Read the model definition and answer for the solid it produces. Units are mm, in the model's axes. A direction names the side the tool comes from. Coordinates: 2 decimals unless noted, no trailing zeros. Write each loop counter-clockwise with the first axis right and the second up, starting at its lowest first coordinate (ties: lowest second). Pieces come first, ordered by that corner, then holes. Notation, with made-up numbers: (22, 11.25) -> (76, 11.25) arc R18 cw to (76, 32.25) -> close; hole circle Ø11 at (35.5, 32). An arc over 180 degrees is marked (long way). Use CSV: the item, a comma, the result in double quotes.
from build123d import *

# Parameters (mm, degrees)
F0_W           = 400
F0_H           = 400
F1_DEPTH       = 50
F2_R           = 6
F3_DEPTH       = 35
F5_D           = 17
F5_DEPTH       = 53
F5_CBORE_D     = 28
F5_CBORE_DEPTH = 20


with BuildPart() as f1:
    # F0 (on Top) → F1 (new body)
    with BuildSketch(Plane.XY):
        Rectangle(F0_W, F0_H)
    extrude(amount=-F1_DEPTH)

    # F2 (on face) → F3 (cut)
    with BuildSketch(Plane.XY):
        with Locations((145, 145)):
            Circle(F2_R)
        with Locations((145, -145)):
            Circle(F2_R)
        with Locations((-145, 145)):
            Circle(F2_R)
        with Locations((-145, -145)):
            Circle(F2_R)
    extrude(amount=-F3_DEPTH, mode=Mode.SUBTRACT)

    # F5
    with Locations(Plane.XY):
        with Locations((160, 92.5), (160, -92.5), (-160, -92.5), (-160, 92.5)):
            CounterBoreHole(F5_D / 2, F5_CBORE_D / 2, F5_CBORE_DEPTH, depth=F5_DEPTH)


solid = f1.part
1. For a pull along Y with two mould halves and no side action, classify faces 1 (the flat face through (-3, 200, -25)), 2 (the flat face through (-200, -3, -25)), 3 (the flat face through (-154, -99, -20)) as pulls with the +Y half, pulls with the -Y half, needs draft (parallel to the pull), parting line crosses it, or undercut.
Solutions:
face 1,"pulls with the +Y half"
face 2,"needs draft"
face 3,"undercut"
2. A cutting plane is placed at B-B (x = -160). Give the vertices of the cut face in (y, z), and give its area (3 significant figures).
Solutions:
outline,"(-200, -50) -> (-101, -50) -> (-101, -20) -> (-106.5, -20) -> (-106.5, 0) -> (-200, 0) -> close; (-84, -50) -> (84, -50) -> (84, -20) -> (78.5, -20) -> (78.5, 0) -> (-78.5, 0) -> (-78.5, -20) -> (-84, -20) -> close; (101, -50) -> (200, -50) -> (200, 0) -> (106.5, 0) -> (106.5, -20) -> (101, -20) -> close"
area,"17,900 mm^2"
3. Find the intervals of material crossed by line 1 along Y through (x, z) = (-145, -22); line 2 along Y through (x, z) = (160, -6.25); line 3 along X through (y, z) = (99.5, -48), in increasing order.
Solutions:
line 1,"y = -200 to -151, -139 to 139, 151 to 200"
line 2,"y = -200 to -106.5, -78.5 to 78.5, 106.5 to 200"
line 3,"x = -200 to -164.82, -155.18 to 155.18, 164.82 to 200"
4. A cutting plane is placed at D-D (y = -145). Give the vertices of the cut face in (x, z), and give its area (3 significant figures).
Solutions:
outline,"(-200, -50) -> (200, -50) -> (200, 0) -> (151, 0) -> (151, -35) -> (139, -35) -> (139, 0) -> (-139, 0) -> (-139, -35) -> (-151, -35) -> (-151, 0) -> (-200, 0) -> close"
area,"19,200 mm^2"
5. A cutting plane is placed at C-C (y = -92.5). Give the vertices of the cut face in (x, z).
Solutions:
outline,"(-200, -50) -> (-168.5, -50) -> (-168.5, -20) -> (-174, -20) -> (-174, 0) -> (-200, 0) -> close; (-151.5, -50) -> (151.5, -50) -> (151.5, -20) -> (146, -20) -> (146, 0) -> (-146, 0) -> (-146, -20) -> (-151.5, -20) -> close; (168.5, -50) -> (200, -50) -> (200, 0) -> (174, 0) -> (174, -20) -> (168.5, -20) -> close"
6. A tool of negligible diameter and unlimited length cuts with its end or side. For faces 4 (the flat face through (-154, 86, -20)), 5 (the flat face through (-3, 3, 0)), from which of +Z, -Z, +X, -X, +Y, -Y can it reach the whole face along a straight path? Write none if from no direction.
Solutions:
face 4,"+Z"
face 5,"+Z, +X, -X, +Y, -Y"
7. A cutting plane is placed at A-A (z = -15). Give the number of separate pieces and of enclosed holes in the cut face, and give its area (3 significant figures).
Solutions:
separate pieces,"1"
enclosed holes,"8"
area,"157,000 mm^2"
8. Each of these flat-tipped pins is pushed along its axis until it touches: pin 1 Ø22 at (x, y) = (-160, -92.5) entering from +Z; pin 2 Ø3 at (x, y) = (129.5, -35.5) entering from +Z; pin 3 Ø9.5 at (x, y) = (-145, 145) entering from +Z; pin 4 Ø15.5 at (x, y) = (-160, 92.5) entering from -Z. Where does it stop, or does it pass through?
Solutions:
pin 1,"stops at z = -20"
pin 2,"stops at z = 0"
pin 3,"stops at z = -35"
pin 4,"passes through"
